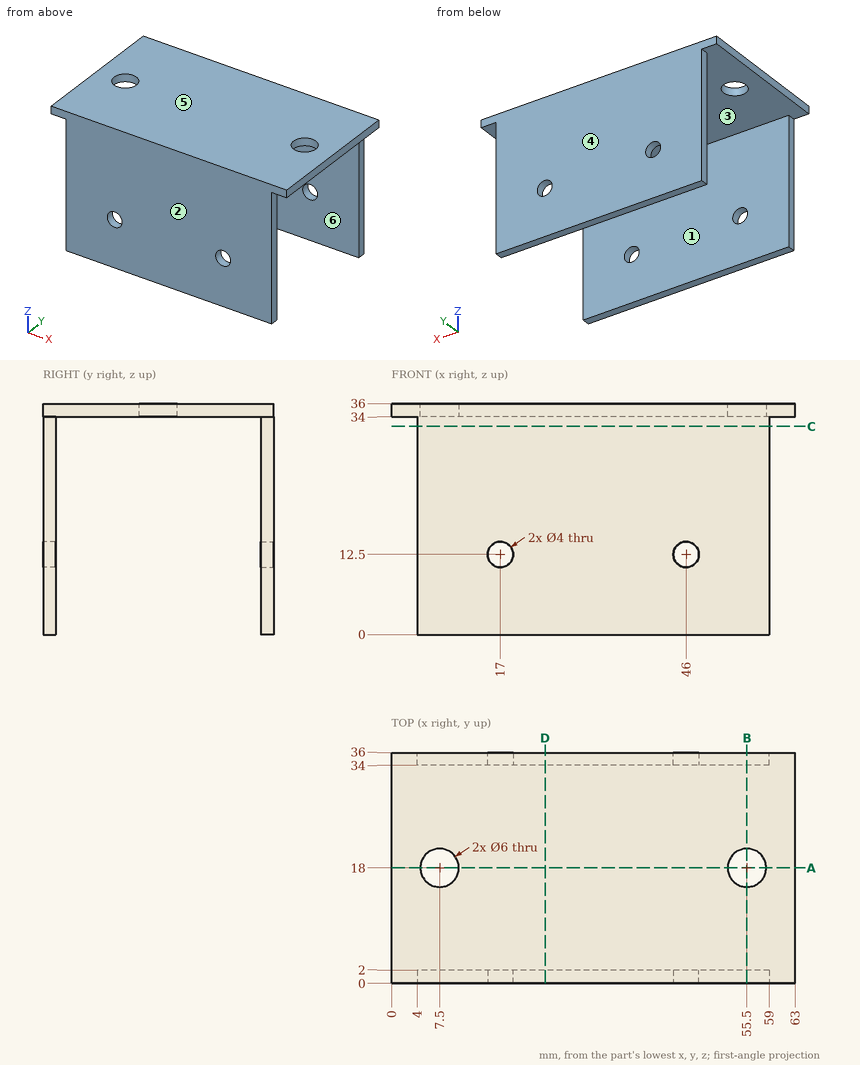
Check sheet for the drawn part. Datum: minimum x, y, z corner. Units: mm. A direction names the side the tool comes from. Round coordinates to 2 decimals unless told otherwise and drop trailing zeros. Order: outer loops, then holes, each group sorted by start corner. A loop starts at its lowest first (then second) coordinate and runs counter-clockwise, first axis right, second up. Notation, with made-up numbers: (34, -0.5) -> (78, -0.5) arc R9 ccw to (78, 8.5) -> close; hole circle Ø5 at (61.5, -12.75). An arc over 180 degrees is marked (long way). Put each result on its own line as item: value.
1) Section check A-A (y = 18). Record the cut outline in (x, z).
Final values:
outline: (0, 34) -> (4.5, 34) -> (4.5, 36) -> (0, 36) -> close; (10.5, 34) -> (52.5, 34) -> (52.5, 36) -> (10.5, 36) -> close; (58.5, 34) -> (63, 34) -> (63, 36) -> (58.5, 36) -> close
2) Depth check by flat-ended pin: pin 1 (4.5 mm diameter, centred on x = 17, z = 12.5, fed in from -Y); pin 2 (1.6 mm diameter, centred on y = 35, z = 15, fed in from -X); pin 3 (0.6 mm diameter, centred on y = 1, z = 11.5, fed in from +X); pin 4 (6 mm diameter, centred on x = 54, y = 19, fed in from -Z). Enter the tip coordinate at first touch or a pass-through.
Final values:
pin 1: stops at y = 0
pin 2: stops at x = 4
pin 3: stops at x = 59
pin 4: stops at z = 34
3) Material ranges on line 1 (X direction, y = 34.5, z = 12.5); line 2 (Y direction, x = 27, z = 28); line 3 (Y direction, x = 55.5, z = 35.05), recorded low to high.
Final values:
line 1: x = 4 to 15, 19 to 44, 48 to 59
line 2: y = 0 to 2, 34 to 36
line 3: y = 0 to 15, 21 to 36
4) Mould release check, pull along Y, two halves, no side actions. Record for the marked faces 1, 2, 3 and 4: +Y half, -Y half, draft (parallel to the pull), parting line (faces both ways), or undercut.
Final values:
face 1: undercut
face 2: -Y half
face 3: undercut
face 4: +Y half
5) Set-up check for the marked faces 5 and 6: record each of +Z, -Z, +X, -X, +Y, -Y from which the full face is reachable in a straight line by a thin tool's end or side.
Final values:
face 5: +Z, +X, -X, +Y, -Y
face 6: -Z, +X, -X
6) Section check C-C (z = 32.5). Record the cut outline in (x, y).
Final values:
outline: (4, 0) -> (59, 0) -> (59, 2) -> (4, 2) -> close; (4, 34) -> (59, 34) -> (59, 36) -> (4, 36) -> close
7) Section check B-B (x = 55.5). Record the cut outline in (y, z).
Final values:
outline: (0, 0) -> (2, 0) -> (2, 34) -> (15, 34) -> (15, 36) -> (0, 36) -> close; (21, 34) -> (34, 34) -> (34, 0) -> (36, 0) -> (36, 36) -> (21, 36) -> close
8) Section check D-D (x = 24). Record the cut outline in (y, z), then the cut area to 3 significant figures.
Final values:
outline: (0, 0) -> (2, 0) -> (2, 34) -> (34, 34) -> (34, 0) -> (36, 0) -> (36, 36) -> (0, 36) -> close
area: 208 mm^2
